Could you check a few things on this model? Use its own coordinates, in mm. A direction names the side the tool comes from. Round coordinates to 2 decimals unless told otherwise and drop trailing zeros. Loops run counter-clockwise (first coordinate to the right, second up) from the corner with the lowest first, then second, coordinate; pieces in that order, holes last. Notation, with made-up numbers: (24, -35.75) -> (83, -35.75) arc R19 ccw to (83, -13.75) -> close; hole circle Ø2 at (-21.75, -14). An arc over 180 degrees is marked (long way). Use CSV: the item, a comma, the result in double quotes. Start each with the question number.
```python
from build123d import *

# Parameters (mm, degrees)
SKETCH1_W          = 141.75
SKETCH1_H          = 57.45
SKETCH1_R          = 2
PLATE2BASE_DEPTH   = 4
SKETCH3_W          = 10
SKETCH3_H          = 57.45
PIBASE_DEPTH       = 4
SKETCH4_R          = 3
PIMOUNT_DEPTH      = 22
SKETCH5_R          = 2
CUT_EXTRUDE2_DEPTH = 4
SKETCH6_R          = 2
CAMMOUNT_DEPTH     = 4


with BuildPart() as part:
    # Sketch1 → Plate2BAse (new body)
    with BuildSketch(Plane(origin=(0, 0, 0), x_dir=(1, 0, 0), z_dir=(0, 1, 0))):
        with Locations((-36.26925, -9.048375)):
            Rectangle(SKETCH1_W, SKETCH1_H)
        with Locations(Location((-102.14425, 14.676625, 0), (0, 0, 270))):
            Circle(SKETCH1_R, mode=Mode.SUBTRACT)
        with Locations(Location((-68.64425, 14.676625, 0), (0, 0, 270))):
            Circle(SKETCH1_R, mode=Mode.SUBTRACT)
        with Locations(Location((-68.64425, 4.676625, 0), (0, 0, 270))):
            Circle(SKETCH1_R, mode=Mode.SUBTRACT)
        with Locations(Location((-102.14425, 4.676625, 0), (0, 0, 270))):
            Circle(SKETCH1_R, mode=Mode.SUBTRACT)
        with Locations(Location((-102.14425, -22.773375, 0), (0, 0, 90))):
            Circle(SKETCH1_R, mode=Mode.SUBTRACT)
        with Locations(Location((-68.64425, -32.773375, 0), (0, 0, 90))):
            Circle(SKETCH1_R, mode=Mode.SUBTRACT)
        with Locations(Location((-68.64425, -22.773375, 0), (0, 0, 90))):
            Circle(SKETCH1_R, mode=Mode.SUBTRACT)
        with Locations(Location((-102.14425, -32.773375, 0), (0, 0, 90))):
            Circle(SKETCH1_R, mode=Mode.SUBTRACT)
    extrude(amount=PLATE2BASE_DEPTH)

    # Sketch3 → PiBase (add)
    with BuildSketch(Plane(origin=(0, 4, 0), x_dir=(1, 0, 0), z_dir=(0, 1, 0))):
        with Locations((-88.955971023, -9.048375)):
            Rectangle(SKETCH3_W, SKETCH3_H)
        with Locations((-12.955971023, -9.048375)):
            Rectangle(SKETCH3_W, SKETCH3_H)
    extrude(amount=PIBASE_DEPTH)

    # Sketch4 → PiMount (cut)
    with BuildSketch(Plane(origin=(0, 8, 0), x_dir=(1, 0, 0), z_dir=(0, 1, 0))):
        with Locations(Location((-12.955971023, 15.201625, 0), (0, 0, 270))):
            Circle(SKETCH4_R)
        with Locations(Location((-12.955971023, -33.298375, 0), (0, 0, 270))):
            Circle(SKETCH4_R)
    extrude(amount=-PIMOUNT_DEPTH, mode=Mode.SUBTRACT)

    # Sketch5 → Cut-Extrude2 (cut)
    with BuildSketch(Plane(origin=(0, 4, 0), x_dir=(1, 0, 0), z_dir=(0, 1, 0))):
        with Locations(Location((-2.955971023, 14.676625, 0), (0, 0, 270))):
            Circle(SKETCH5_R)
        with Locations(Location((7.044028977, 14.676625, 0), (0, 0, 270))):
            Circle(SKETCH5_R)
        with Locations(Location((17.044028977, 14.676625, 0), (0, 0, 270))):
            Circle(SKETCH5_R)
        with Locations(Location((27.044028977, 14.676625, 0), (0, 0, 270))):
            Circle(SKETCH5_R)
        with Locations(Location((7.044028977, 4.676625, 0), (0, 0, 270))):
            Circle(SKETCH5_R)
        with Locations(Location((17.044028977, 4.676625, 0), (0, 0, 270))):
            Circle(SKETCH5_R)
        with Locations(Location((27.044028977, 4.676625, 0), (0, 0, 270))):
            Circle(SKETCH5_R)
        with Locations(Location((-2.955971023, 4.676625, 0), (0, 0, 270))):
            Circle(SKETCH5_R)
        with Locations(Location((-2.955971023, -22.773375, 0), (0, 0, 90))):
            Circle(SKETCH5_R)
        with Locations(Location((27.044028977, -22.773375, 0), (0, 0, 90))):
            Circle(SKETCH5_R)
        with Locations(Location((17.044028977, -22.773375, 0), (0, 0, 90))):
            Circle(SKETCH5_R)
        with Locations(Location((7.044028977, -22.773375, 0), (0, 0, 90))):
            Circle(SKETCH5_R)
        with Locations(Location((27.044028977, -32.773375, 0), (0, 0, 90))):
            Circle(SKETCH5_R)
        with Locations(Location((17.044028977, -32.773375, 0), (0, 0, 90))):
            Circle(SKETCH5_R)
        with Locations(Location((7.044028977, -32.773375, 0), (0, 0, 90))):
            Circle(SKETCH5_R)
        with Locations(Location((-2.955971023, -32.773375, 0), (0, 0, 90))):
            Circle(SKETCH5_R)
        with Locations(Location((-2.955971023, -9.048375, 0), (0, 0, 270))):
            Circle(SKETCH5_R)
        with Locations(Location((7.044028977, -9.048375, 0), (0, 0, 270))):
            Circle(SKETCH5_R)
        with Locations(Location((17.044028977, -9.048375, 0), (0, 0, 270))):
            Circle(SKETCH5_R)
        with Locations(Location((27.044028977, -9.048375, 0), (0, 0, 270))):
            Circle(SKETCH5_R)
    extrude(amount=-CUT_EXTRUDE2_DEPTH, mode=Mode.SUBTRACT)

    # Sketch6 → CamMount (cut)
    with BuildSketch(Plane(origin=(0, 4, 0), x_dir=(1, 0, 0), z_dir=(0, 1, 0))):
        with Locations(Location((-102.14425, -4.048375, 0), (0, 0, 270))):
            Circle(SKETCH6_R)
        with Locations(Location((-102.14425, -14.048375, 0), (0, 0, 90))):
            Circle(SKETCH6_R)
    extrude(amount=-CAMMOUNT_DEPTH, mode=Mode.SUBTRACT)


solid = part.part
```
1. Will these pins go through, and if not, where does the flat tip stop? pin 1 (10 mm diameter, centred on x = 20, z = 26, fed in from +Y); pin 2 (5.5 mm diameter, centred on x = -12.96, z = 33.3, fed in from +Y).
2. If I drill on L1, parallel to X at y = 0.5, z = 9; L2, parallel to X at y = 7, z = -10; L3, parallel to Y at x = 6, z = 25, over which ranges is the centre line in solid material (lowest first)?
3. For faces 1 (the face through (-7.956, 6, 9)), 2 (the face through (-17.956, 6, 9)), 3 (the face through (15.09, 2.03, -15.11)), which set-ups out of +Z, -Z, +X, -X, +Y, -Y let a thin tool reach every point of the face, with its end or its side?
4. We'd pull the mould along Z, two halves only. Please class faces 4 (the face through (7.81, 2.028, 30.926)), 5 (the face through (-37, 2, -19.677)), 6 (the face through (-51, 4, 9)): pulls with the +Z half, pulls with the -Z half, needs draft (parallel to the pull), parting line crosses it, or undercut.
5. Suppose I cut it at A-A (y = 5.5). List the corners of the cut face in (x, z) for me.
6. Suppose I cut it at B-B (z = -10). List the corners of the cut face in (x, y) for me, then the cut area to 3 significant figures.
7. Suppose I cut it at C-C (x = -74.5). List the corners of the cut face in (y, z) for me, then the cut area to 3 significant figures.
Geometry check:
1,pin 1,"stops at y = 4"
1,pin 2,"passes through"
2,L1,"x = -107.14 to -4.96, -0.96 to 5.04, 9.04 to 15.04, 19.04 to 25.04, 29.04 to 34.61"
2,L2,"x = -93.96 to -83.96, -17.96 to -7.96"
2,L3,"y = 0 to 4"
3,face 1,"+Z, -Z, +X, +Y"
3,face 2,"+Z, -Z, +Y"
3,face 3,"+Y, -Y"
4,face 4,"undercut"
4,face 5,"pulls with the -Z half"
4,face 6,"needs draft"
5,outline,"(-93.96, -19.68) -> (-83.96, -19.68) -> (-83.96, 37.77) -> (-93.96, 37.77) -> close; (-17.96, -19.68) -> (-7.96, -19.68) -> (-7.96, 37.77) -> (-17.96, 37.77) -> close; hole circle Ø6 at (-12.96, -15.2); hole circle Ø6 at (-12.96, 33.3)"
6,outline,"(-107.14, 0) -> (34.61, 0) -> (34.61, 4) -> (-7.96, 4) -> (-7.96, 8) -> (-17.96, 8) -> (-17.96, 4) -> (-83.96, 4) -> (-83.96, 8) -> (-93.96, 8) -> (-93.96, 4) -> (-107.14, 4) -> close"
6,area,"647 mm²"
7,outline,"(0, -19.68) -> (4, -19.68) -> (4, 37.77) -> (0, 37.77) -> close"
7,area,"230 mm²"
